Autodesk Inventor part; units mm, degrees
ref_plane "YZ Plane" through (0, 0, 0) normal (1, 0, 0) x (0, 1, 0)
ref_plane "XZ Plane" through (0, 0, 0) normal (0, 1, 0) x (-1, 0, 0)
ref_plane "XY Plane" through (0, 0, 0) normal (0, 0, 1) x (1, 0, 0)
sketch "Boceto1" plane through (0, 0, 0) normal (0, 1, 0) x (-1, 0, 0)
  line L0 (54, 60) -> (-54, 60)
  line L1 (-54, 60) -> (-54, -60)
  line L2 (-54, -60) -> (54, -60)
  line L3 (54, -60) -> (54, 60)
  line L4 (141.1986, 0) -> (-141.1986, 0) construction
  line L5 (0, -44.0939) -> (0, 44.0939) construction
  point P0 (0, 0)
  point P1 (54, 0)
  point P2 (0, -60)
  point P3 (0, 0)
  dimension "d0" = 108
  dimension "d1" = 120
extrude "Extrusión1" add sketch "Boceto1" along normal blind 4
sketch "Boceto2" plane through (0, 4, 0) normal (0, 1, 0) x (1, 0, 0)
  circle A0 centre (-46.5, 36.3333) radius 1.5
  circle A1 centre (-3.5, 36.3333) radius 1.5
  circle A2 centre (-46.5, -31.6667) radius 1.5
  circle A3 centre (-3.5, -31.6667) radius 1.5
  circle A4 centre (4.25, -14.9167) radius 1.5
  circle A5 centre (46.75, -14.9167) radius 1.5
  circle A6 centre (46.75, 23.5833) radius 1.5
  circle A7 centre (4.25, 23.5833) radius 1.5
  circle A8 centre (0, -50) radius 1.5
  circle A9 centre (28, -50) radius 1.5
  circle A10 centre (-28, -50) radius 1.5
  line L0 (-28, -50) -> (28, -50) construction
  line L1 (-54, -60) -> (54, -60) construction
  circle A11 centre (-46.5, 36.3333) radius 7
  circle A12 centre (-3.5, 36.3333) radius 7
  circle A13 centre (4.25, 23.5833) radius 7
  circle A14 centre (46.75, 23.5833) radius 7
  circle A15 centre (46.75, -14.9167) radius 7
  circle A16 centre (4.25, -14.9167) radius 7
  circle A17 centre (-3.5, -31.6667) radius 7
  circle A18 centre (-46.5, -31.6667) radius 7
  circle A19 centre (-28, -50) radius 7
  circle A20 centre (0, -50) radius 7
  circle A21 centre (28, -50) radius 7
  point P0 (0, 0)
  dimension "d9" = 28
  dimension "d10" = 3
  dimension "d11" = 10
  dimension "d33" = 14
sketch "Boceto3" plane through (0, 4, 0) normal (0, 1, 0) x (1, 0, 0)
  line L0 (-54, -60) -> (54, -60)
  line L1 (54, -60) -> (54, 60)
  line L2 (54, 60) -> (-54, 60)
  line L3 (-54, 60) -> (-54, -60)
  line L4 (-42, 48) -> (42, 48)
  line L5 (42, 48) -> (42, -48)
  line L6 (42, -48) -> (-42, -48)
  line L7 (-42, -48) -> (-42, 48)
  line L8 (-42, 36.6863) -> (-30.6863, 48)
  line L9 (-42, 25.3726) -> (-19.3726, 48)
  line L10 (-42, 14.0589) -> (-8.0589, 48)
  line L11 (-42, 2.7452) -> (3.2548, 48)
  line L12 (-42, -8.5685) -> (14.5685, 48)
  line L13 (-42, -19.8823) -> (25.8823, 48)
  line L14 (-42, -31.196) -> (37.196, 48)
  line L15 (-42, -42.5097) -> (42, 41.4903)
  line L16 (-36.1766, -48) -> (42, 30.1766)
  line L17 (-24.8629, -48) -> (42, 18.8629)
  line L18 (-13.5492, -48) -> (42, 7.5492)
  line L19 (-2.2355, -48) -> (42, -3.7645)
  line L20 (9.0782, -48) -> (42, -15.0782)
  line L21 (20.3919, -48) -> (42, -26.3919)
  line L22 (31.7056, -48) -> (42, -37.7056)
  point P0 (0, 0)
  point P1 (0, 48)
  point P2 (0, 60)
  dimension "d12" = 12
  dimension "d13" = 12
  dimension "d14" = 12
  dimension "d15" = 45
  dimension "d16" = 8
  dimension "d17" = 8
  dimension "d18" = 8
  dimension "d19" = 8
  dimension "d20" = 8
  dimension "d21" = 8
  dimension "d22" = 8
  dimension "d23" = 8
  dimension "d24" = 8
  dimension "d25" = 8
  dimension "d26" = 8
  dimension "d27" = 8
  dimension "d28" = 8
  dimension "d29" = 8
  dimension "d30" = 8
extrude "Extrusión2" cut sketch "Boceto3" against normal blind 10 contours L4 L8 L7 | L4 L10 L7 L9 | L4 L12 L7 L11 | L4 L14 L7 L13 | L15 L5 L16 L6 L7 | L5 L18 L6 L17 | L5 L20 L6 L19 | L5 L22 L6 L21
extrude "Extrusión3" add sketch "Boceto2" against normal blind 4
sketch "Boceto4" plane through (0, 4, 0) normal (0, 1, 0) x (1, 0, 0)
  circle A0 centre (-46.5, 36.3333) radius 1.5
  circle A1 centre (46.75, 23.5833) radius 1.5
  circle A2 centre (46.75, -14.9167) radius 1.5
  circle A3 centre (28, -50) radius 1.5
  circle A4 centre (0, -50) radius 1.5
  circle A5 centre (-28, -50) radius 1.5
  circle A6 centre (-46.5, -31.6667) radius 1.5
  circle A7 centre (4.25, -14.9167) radius 1.5
  point P0 (0, 0)
extrude "Extrusión4" cut sketch "Boceto4" against normal through all
sketch "Boceto5" plane through (0, 4, 0) normal (0, 1, 0) x (1, 0, 0)
  circle A0 centre (-46.1942, 50) radius 1.5
  circle A1 centre (47.5275, 50) radius 1.5
  circle A2 centre (-46.1942, -50) radius 1.5
  circle A3 centre (47.5275, -50) radius 1.5
  point P0 (0, 0)
extrude "Extrusión5" cut sketch "Boceto5" against normal through all
equation "\"d13\" = d12"
equation "\"d18\" = d16"
equation "\"d19\" = d18"
equation "\"d20\" = d19"
equation "\"d21\" = d20"
equation "\"d22\" = d21"
equation "\"d23\" = d22"
equation "\"d24\" = d23"
equation "\"d25\" = d24"
equation "\"d26\" = d25"
equation "\"d27\" = d26"
equation "\"d28\" = d27"
equation "\"d29\" = d28"
equation "\"d30\" = d29"
properties part number "bandeja componentes"
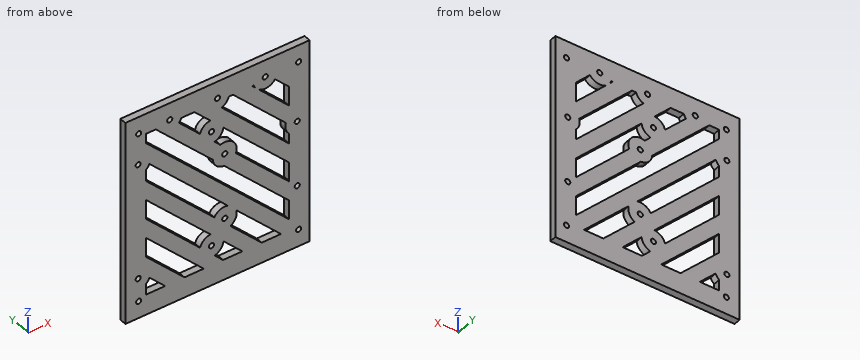
Can you work these out from the model? Positions are in its coordinate system, mm. Coordinates: 2 decimals unless noted, no trailing zeros. Write each loop counter-clockwise with the first axis right and the second up, starting at its lowest first coordinate (ties: lowest second). Pieces come first, ordered by that corner, then holes. Notation, with made-up numbers: (85, 41.5) -> (110, 41.5) arc R22 ccw to (110, 60.5) -> close; hole circle Ø11 at (14, 34.5). An arc over 180 degrees is marked (long way). Write each question's results on one line, items separated by ' | '. Start each with the question number.
Item 1: If we section it at B-B, the plane x = -32: Write out the boundary of the cut face in (y, z), and give its area (3 significant figures).
Item 2: If we section it at D-D, the plane z = -27.5: Write out the boundary of the cut face in (x, y).
Item 3: If we section it at A-A, the plane z = 50: Write out the boundary of the cut face in (x, y), and give its area (3 significant figures).
Item 4: Please list where these lines run through material, in increasing order: probe 1 along X at (y, z) = (2, -50); probe 2 along X at (y, z) = (3.1, 50); probe 3 along Z at (x, y) = (-13.5, 0.55).
Item 5: If we section it at C-C, the plane x = 18.5: Write out the boundary of the cut face in (y, z).
Answer block:
1) outline: (0, -60) -> (4, -60) -> (4, -48) -> (0, -48) -> close; (0, -46.69) -> (4, -46.69) -> (4, -35.37) -> (0, -35.37) -> close; (0, -24.06) -> (4, -24.06) -> (4, -12.75) -> (0, -12.75) -> close; (0, -1.43) -> (4, -1.43) -> (4, 9.88) -> (0, 9.88) -> close; (0, 21.2) -> (4, 21.2) -> (4, 32.51) -> (0, 32.51) -> close; (0, 43.82) -> (4, 43.82) -> (4, 60) -> (0, 60) -> close | area: 294 mm²
2) outline: (-54, 0) -> (-39.87, 0) -> (-39.87, 4) -> (-54, 4) -> close; (-28.56, 0) -> (-17.25, 0) -> (-17.25, 4) -> (-28.56, 4) -> close; (-5.93, 0) -> (10.05, 0) -> (10.05, 4) -> (-5.93, 4) -> close; (16.7, 0) -> (28.01, 0) -> (28.01, 4) -> (16.7, 4) -> close; (39.32, 0) -> (54, 0) -> (54, 4) -> (39.32, 4) -> close
3) outline: (-54, 0) -> (-47.69, 0) -> (-47.69, 4) -> (-54, 4) -> close; (-44.69, 0) -> (-29.5, 0) -> (-29.5, 4) -> (-44.69, 4) -> close; (-26.5, 0) -> (-1.5, 0) -> (-1.5, 4) -> (-26.5, 4) -> close; (1.5, 0) -> (26.5, 0) -> (26.5, 4) -> (1.5, 4) -> close; (29.5, 0) -> (46.03, 0) -> (46.03, 4) -> (29.5, 4) -> close; (49.03, 0) -> (54, 0) -> (54, 4) -> (49.03, 4) -> close | area: 372 mm²
4) probe 1: -54 to -47.69, -44.69 to 46.03, 49.03 to 54 | probe 2: -54 to -47.69, -44.69 to -29.5, -26.5 to -1.5, 1.5 to 26.5, 29.5 to 46.03, 49.03 to 54 | probe 3: -60 to -48, -42.56 to -31.25, -19.93 to -8.62, 2.7 to 14.01, 25.32 to 36.64, 47.95 to 60
5) outline: (0, -60) -> (4, -60) -> (4, -40.62) -> (0, -40.62) -> close; (0, -29.3) -> (4, -29.3) -> (4, -17.99) -> (0, -17.99) -> close; (0, -6.68) -> (4, -6.68) -> (4, 4.64) -> (0, 4.64) -> close; (0, 15.95) -> (4, 15.95) -> (4, 27.26) -> (0, 27.26) -> close; (0, 38.58) -> (4, 38.58) -> (4, 60) -> (0, 60) -> close
